Geometry check sheet. Reference: the model listing, model coordinates, mm. Face numbers are marked on the shaded views. Give positions to 0.01 mm unless a question says otherwise; leave off trailing zeros. Loops run counter-clockwise (first coordinate to the right, second up) from the corner with the lowest first, then second, coordinate; pieces in that order, holes last. Notation, with made-up numbers: (12, 20) -> (31, 20) arc R10 cw to (31, 38) -> close; hole circle Ø9 at (5.5, -20.5). An arc over 180 degrees is marked (long way). One line per question, with ' | ' between items.
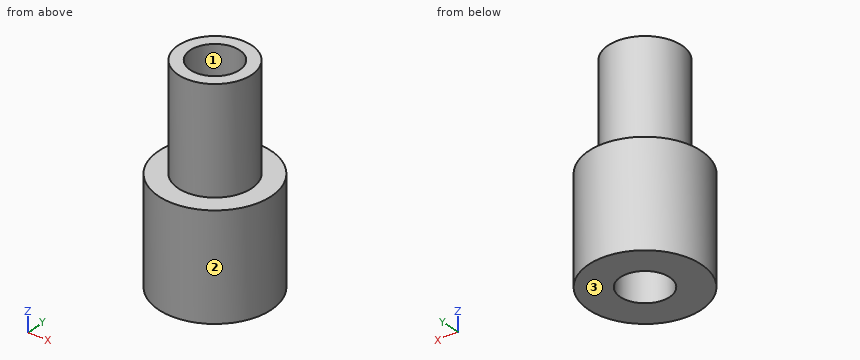
from build123d import *

# Parameters (mm, degrees)
F0_R     = 26.964837
F1_DEPTH = 50
F2_R     = 17.581895
F3_DEPTH = 50
F4_R     = 11.797874
F5_DEPTH = 100.001


with BuildPart() as f1:
    # F0 (on Top) → F1 (new body)
    with BuildSketch(Plane.XY):
        Circle(F0_R)
    extrude(amount=F1_DEPTH)

    # F2 (on face) → F3 (join)
    with BuildSketch(Plane.XY.offset(50)):
        Circle(F2_R)
    extrude(amount=F3_DEPTH)

    # F4 (on face) → F5 (cut, through all)
    with BuildSketch(Plane.XY.offset(100)):
        Circle(F4_R)
    extrude(amount=-F5_DEPTH, mode=Mode.SUBTRACT)


solid = f1.part
Item 1: Sectioned sample at A-A (y = 0). Record the cut outline in (x, z).
Result:
outline: (-26.96, 0) -> (-11.8, 0) -> (-11.8, 100) -> (-17.58, 100) -> (-17.58, 50) -> (-26.96, 50) -> close; (11.8, 0) -> (26.96, 0) -> (26.96, 50) -> (17.58, 50) -> (17.58, 100) -> (11.8, 100) -> close
Item 2: Scan lines: probe 1 along Y at (x, z) = (0, 69); probe 2 along Y at (x, z) = (0, 31); probe 3 along Z at (x, y) = (11.5, 14). Record each from-to range of solid material in increasing order.
Result:
probe 1: -17.58 to -11.8, 11.8 to 17.58 | probe 2: -26.96 to -11.8, 11.8 to 26.96 | probe 3: 0 to 50
Item 3: Depth check by flat-ended pin: pin 1 Ø1.5 at (x, z) = (13, 30.5) entering from +Y; pin 2 Ø2 at (x, z) = (8, 33) entering from +Y; pin 3 Ø2 at (x, z) = (-9.5, 71) entering from +Y. Enter the tip coordinate at first touch or a pass-through.
Result:
pin 1: y = 24.02 | pin 2: y = 26.04 | pin 3: y = 15.39
Item 4: Sectioned sample at D-D (z = 18). Record the cut outline in (x, y).
Result:
outline: circle Ø53.93 at (0, 0); hole circle Ø23.6 at (0, 0)
Item 5: Release check for a two-part mould opening along Y. For the marked faces 1, 2 and 3 record: pulls with the +Y half, pulls with the -Y half, needs draft (parallel to the pull), parting line crosses it, or undercut.
Result:
face 1: undercut | face 2: parting line crosses it | face 3: needs draft
Item 6: Sectioned sample at C-C (x = 14.5). Record the cut outline in (y, z).
Result:
outline: (-22.73, 0) -> (22.73, 0) -> (22.73, 50) -> (9.94, 50) -> (9.94, 100) -> (-9.94, 100) -> (-9.94, 50) -> (-22.73, 50) -> close
